The figure shows three views and two pictorial views of one solid part (mm, origin at its lowest corner). Answer the questions. Round coordinates to 2 decimals unless told otherwise and drop trailing zeros. Order: outer loops, then holes, each group sorted by start corner. A loop starts at its lowest first (then second) coordinate and runs counter-clockwise, first axis right, second up. Notation, with made-up numbers: (75, 68.25) - (115, 68.25) arc R23 cw to (115, 94.25) - close; hole circle Ø5 at (-17, 35). An arc over 180 degrees is marked (long way). Use CSV: the item, a comma, the result in double quotes. Start each with the question number.
Item 1: Flat-ended cylindrical pins translate along their axes: P1, Ø1, axis at x = 76, z = 9.5, coming from the +Y side; P2, Ø2, axis at x = 93, z = 2, coming from the +Y side; P3, Ø6, axis at x = 34, z = 1.5, coming from the +Y side. Find the tip coordinate at first contact, or state that the pin passes through.
Item 2: Find section B-B, the plane y = 67.5. Give the vertices of the cut face in (x, z).
Item 3: Straight lines are drawn through the part: line 1 along Y through (x, z) = (53, 5.5); line 2 along X through (y, z) = (54, 12.75); line 3 along Y through (x, z) = (16.5, 7.75). For each, find the intervals that lie inside material, in ascending order. Write a range as [from, to].
Item 4: Determine the mould class of the marked faces 1 and 2 for opening direction Y: +Y half, -Y half, draft (parallel to the pull), parting line (faces both ways), or undercut.
Item 5: Find section A-A, the plane x = 53. Give the vertices of the cut face in (y, z), plus the area to 3 significant figures.
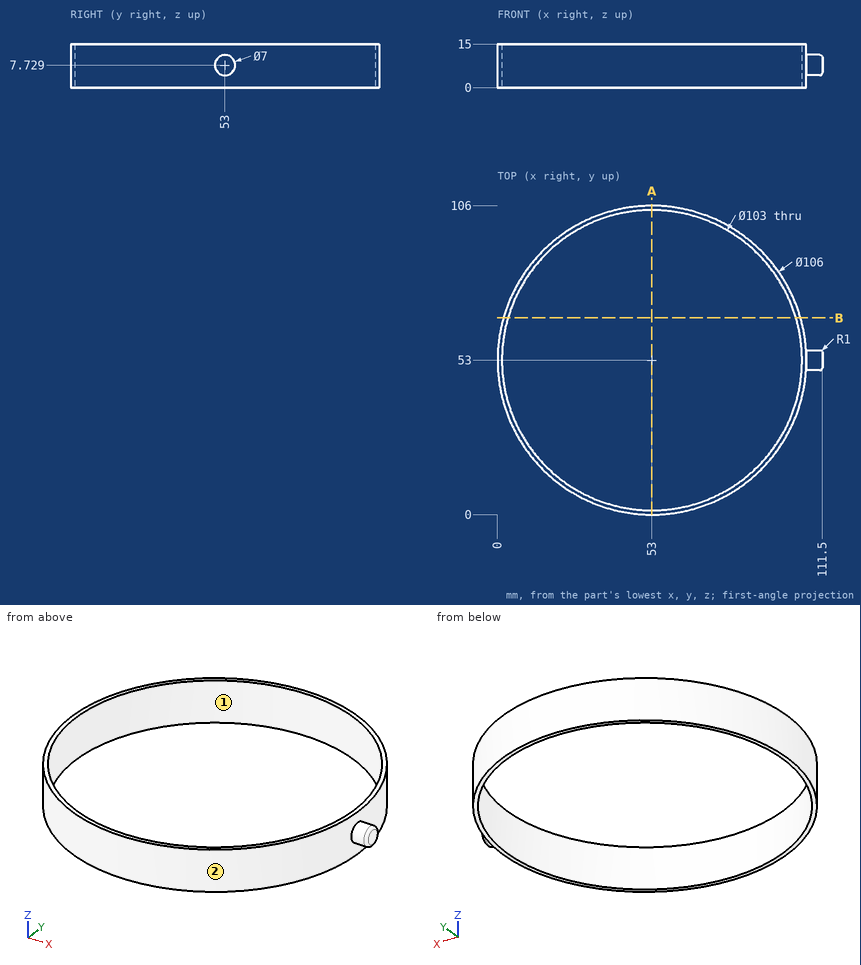
Worked out:
1,P1,"stops at y = 100.99"
1,P2,"stops at y = 88.89"
1,P3,"stops at y = 103.53"
2,outline,"(2.02, 0) - (3.58, 0) - (3.58, 15) - (2.02, 15) - close; (102.42, 0) - (103.98, 0) - (103.98, 15) - (102.42, 15) - close"
3,line 1,"y = [0, 1.5], [104.5, 106]"
3,line 2,"x = [0.01, 1.51], [104.49, 105.99]"
3,line 3,"y = [14.57, 16.67], [89.33, 91.43]"
4,face 1,"undercut"
4,face 2,"parting line"
5,outline,"(0, 0) - (1.5, 0) - (1.5, 15) - (0, 15) - close; (104.5, 0) - (106, 0) - (106, 15) - (104.5, 15) - close"
5,area,"45.0 mm²"
